Can you work these out from the model? Positions are in its coordinate system, mm. A direction names the side the tool comes from. Coordinates: 2 decimals unless noted, no trailing zeros. Order: outer loops, then holes, each group sorted by start corner. A loop starts at its lowest first (then second) coordinate and runs counter-clockwise, first axis right, second up. Notation, with made-up numbers: (-2, -34) -> (10, -34) arc R34 ccw to (10, -1) -> close; hole circle Ø10 at (-27.75, 41.25). An arc over 180 degrees is marked (long way). Write item = value, one per line.
Autodesk Inventor part; units mm, degrees
ref_plane "YZ Plane" through (0, 0, 0) normal (1, 0, 0) x (0, 1, 0)
ref_plane "XZ Plane" through (0, 0, 0) normal (0, 1, 0) x (-1, 0, 0)
ref_plane "XY Plane" through (0, 0, 0) normal (0, 0, 1) x (1, 0, 0)
sketch "Sketch1" plane through (0, 0, 0) normal (0, 0, 1) x (1, 0, 0)
  line L0 (0, 0) -> (12.7, 0)
  line L1 (12.7, 0) -> (12.7, 25.4)
  line L2 (12.7, 25.4) -> (0, 25.4)
  line L3 (0, 25.4) -> (0, 0)
  dimension "d0" = 25.4
  dimension "d1" = 12.7
extrude "Extrusion1" add sketch "Sketch1" along normal blind 1.27
sketch "Sketch2" plane through (0, 0, 1.27) normal (0, 0, 1) x (1, 0, 0)
  line L0 (6.35, -14.9929) -> (6.35, 30.5291) construction
  line L1 (12.7, 0) -> (12.7, 25.4) construction
  line L2 (0, 0) -> (12.7, 0)
  point P0 (6.35, 20.32)
  point P1 (6.35, 7.62)
  dimension "d4" = 6.35
  dimension "d5" = 7.62
  dimension "d6" = 12.7
hole "Hole1" at (6.35, 20.32, 1.27) at (6.35, 7.62, 1.27) direction (0, 0, -1) diameter 3.175 depth 25.4 tip angle 118
sketch "Sketch3" plane through (0, 0, 1.27) normal (0, 0, 1) x (1, 0, 0)
  line L0 (12.7, 0) -> (12.7, 25.4)
  line L1 (0, 0) -> (12.7, 0)
  line L2 (12.7, 0) -> (12.7, 1.27)
  line L3 (12.7, 1.27) -> (0, 1.27)
  line L4 (0, 1.27) -> (0, 0)
  dimension "d14" = 1.27
extrude "Extrusion2" add sketch "Sketch3" along normal blind 19.05
sketch "Sketch4" plane through (0, 0, 0) normal (0, -1, 0) x (1, 0, 0)
  line L0 (6.35, -12.0636) -> (6.35, 31.9717) construction
  line L1 (12.7, 0) -> (12.7, 20.32) construction
  circle A0 centre (6.35, 13.97) radius 1.5875
  line L2 (0, 20.32) -> (12.7, 20.32) construction
  point P0 (0, 0)
  dimension "d17" = 6.35
  dimension "d18" = 3.175
  dimension "d19" = 6.35
extrude "Extrusion3" cut sketch "Sketch4" against normal blind 19.05
properties part number "000204"
Item 1: I'm going to push flat-ended pins straight in: P1, Ø1.5, axis at x = 8.5, z = 18, coming from the +Y side; P2, Ø4, axis at x = 1.5, y = 18, coming from the +Z side; P3, Ø3, axis at x = 6.35, y = 20.32, coming from the -Z side. Where does each tip first touch, or does it pass through?
A:
P1 = 1.27
P2 = 1.27
P3 = through
Item 2: If I drill on probe 1 along Y at (x, z) = (6.35, 0.7); probe 2 along X at (y, z) = (20.32, 0.85); probe 3 along Z at (x, y) = (6.35, 1), over which ranges is the centre line in solid material (lowest first)?
A:
probe_1 = 0 to 6.03, 9.21 to 18.73, 21.91 to 25.4
probe_2 = 0 to 4.76, 7.94 to 12.7
probe_3 = 0 to 12.38, 15.56 to 20.32
Item 3: I want a section at C-C, the plane x = 6. Please give me the cut outline in (y, z), plus the area to 3 significant figures.
A:
outline = (0, 0) -> (6.07, 0) -> (6.07, 1.27) -> (1.27, 1.27) -> (1.27, 12.42) -> (0, 12.42) -> close; (0, 15.52) -> (1.27, 15.52) -> (1.27, 20.32) -> (0, 20.32) -> close; (9.17, 0) -> (18.77, 0) -> (18.77, 1.27) -> (9.17, 1.27) -> close; (21.87, 0) -> (25.4, 0) -> (25.4, 1.27) -> (21.87, 1.27) -> close
area = 44.7 mm2
Item 4: I want a section at A-A, the plane y = 7.62. Please give me the cut outline in (x, z), plus the area to 3 significant figures.
A:
outline = (0, 0) -> (4.76, 0) -> (4.76, 1.27) -> (0, 1.27) -> close; (7.94, 0) -> (12.7, 0) -> (12.7, 1.27) -> (7.94, 1.27) -> close
area = 12.1 mm2
Item 5: For faces 4 (the flat face through (6, 14, 1.27)), 5 (the flat face through (0, 9, 1)), which set-ups out of +Z, -Z, +X, -X, +Y, -Y let a thin tool reach every point of the face, with its end or its side?
A:
face_4 = +Z, +X, -X, +Y
face_5 = +Z, -Z, -X, +Y, -Y
Item 6: If we mould it in two halves opening along Y, with no side actions, what happens to faces 1 (the flat face through (6, 0, 10)), 2 (the flat face through (6, 13, 0)), 3 (the cylindrical face through (7.76, 19.59, 0.63))? For each: pulls with the +Y half, pulls with the -Y half, needs draft (parallel to the pull), parting line crosses it, or undercut.
A:
face_1 = pulls with the -Y half
face_2 = needs draft
face_3 = undercut
Item 7: I want a section at D-D, the plane x = 3.5. Please give me the cut outline in (y, z).
A:
outline = (0, 0) -> (25.4, 0) -> (25.4, 1.27) -> (1.27, 1.27) -> (1.27, 20.32) -> (0, 20.32) -> close
